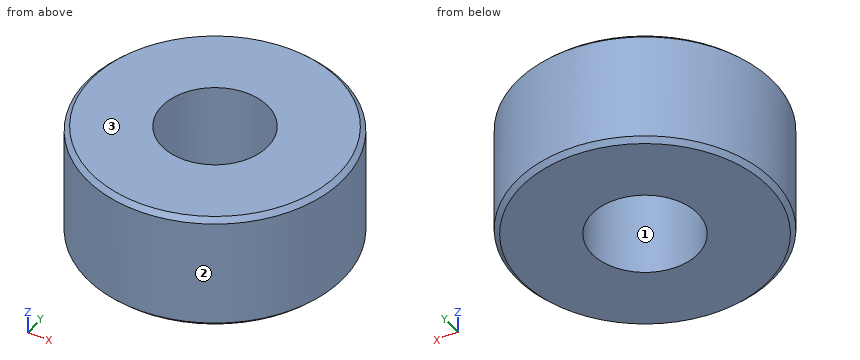
```python
from build123d import *

# Parameters (mm, degrees)
SKETCH1_R               = 27.5
BOSS_EXTRUDE1_DEPTH     = 12.5
CUT_EXTRUDE1_DEPTH      = 41.850336596
CUT_EXTRUDE1_DEPTH_BACK = 41.850336596
SKETCH2_R               = 11.35
CHAMFER1_SIZE           = 1


with BuildPart() as part:
    # Sketch1 → Boss-Extrude1 (new, symmetric)
    with BuildSketch(Plane.XY):
        Circle(SKETCH1_R)
    extrude(amount=BOSS_EXTRUDE1_DEPTH, both=True)

    # Sketch2 → Cut-Extrude1 (cut, two sides: drawn at the far end of the back side and taken through both)
    with BuildSketch(Plane.XY.offset(-CUT_EXTRUDE1_DEPTH_BACK)):
        Circle(SKETCH2_R)
    extrude(amount=CUT_EXTRUDE1_DEPTH + CUT_EXTRUDE1_DEPTH_BACK, mode=Mode.SUBTRACT)

    # Chamfer1
    chamfer1_edges = [part.edges().sort_by_distance(p)[0] for p in [
        (-27.5, 0, -12.5),
        (-27.5, 0, 12.5),
    ]]
    chamfer(chamfer1_edges, length=CHAMFER1_SIZE)


solid = part.part
```
The model under review builds one solid part; all positions refer to its coordinate system, in mm. Face numbers are marked on the shaded views. Coordinates: 2 decimals unless noted, no trailing zeros. Write each loop counter-clockwise with the first axis right and the second up, starting at its lowest first coordinate (ties: lowest second). Pieces come first, ordered by that corner, then holes. Notation, with made-up numbers: (1.25, 75.25) - (18.25, 75.25) arc R18 ccw to (18.25, 110.25) - close; hole circle Ø10 at (-11, 75.25). An arc over 180 degrees is marked (long way). Answer in a Markdown table with one row per item. Add a question column.
Q1. Consider section A-A on x = 0. Give the boundary of the cut face in (y, z), then the cut area to 4 significant figures.
Q2. To check wall thickness, follow line 1 along Y through (x, z) = (0, -3.75); line 2 along X through (y, z) = (9.5, 2.5); line 3 along X through (y, z) = (6, -10.5). State the ranges of each line that lie inside material, in increasing order. Write a range as from..to.
Q3. Consider section C-C on z = -2.75. Give the boundary of the cut face in (x, y), then the cut area to 3 significant figures.
Q4. Clearance check with flat-ended pins moving along their axes: pin 1 (10 mm diameter, centred on y = -6.5, z = -4, fed in from -X); pin 2 (1 mm diameter, centred on y = -11.5, z = -3, fed in from +X); pin 3 (12 mm diameter, centred on x = -1, z = 1.5, fed in from +Y); pin 4 (8 mm diameter, centred on x = 3.5, y = 10.5, fed in from -Z). State where each tip first meets the part, or that it passes through.
Q5. Draft analysis for pull direction Y (two halves, no side actions). For the marked faces 1, 2 and 3, state which applies: +Y half, -Y half, draft (parallel to the pull), parting line (faces both ways), or undercut.
Answers below:
| question | item | result |
|---|---|---|
| 1 | outline | (-27.5, -11.5) - (-26.5, -12.5) - (-11.35, -12.5) - (-11.35, 12.5) - (-26.5, 12.5) - (-27.5, 11.5) - close; (11.35, -12.5) - (26.5, -12.5) - (27.5, -11.5) - (27.5, 11.5) - (26.5, 12.5) - (11.35, 12.5) - close |
| 1 | area | 805.5 mm² |
| 2 | line 1 | -27.5..-11.35, 11.35..27.5 |
| 2 | line 2 | -25.81..-6.21, 6.21..25.81 |
| 2 | line 3 | -26.84..-9.63, 9.63..26.84 |
| 3 | outline | circle Ø55 at (0, 0); hole circle Ø22.7 at (0, 0) |
| 3 | area | 1,970 mm² |
| 4 | pin 1 | x = -27.46 |
| 4 | pin 2 | x = 25.2 |
| 4 | pin 3 | y = 27.5 |
| 4 | pin 4 | z = -12.5 |
| 5 | face 1 | undercut |
| 5 | face 2 | parting line |
| 5 | face 3 | draft |
